Design review of the part built by this model. Coordinates are the model's own, in mm. Face numbers are marked on the shaded views. A direction names the side the tool comes from. Give positions to 0.01 mm unless a question says otherwise; leave off trailing zeros. Loops run counter-clockwise (first coordinate to the right, second up) from the corner with the lowest first, then second, coordinate; pieces in that order, holes last. Notation, with made-up numbers: M 28,34.5 L 57,34.5 A18 cw 57,58.5 Z; hole C 86.25,20.25 d4. An arc over 180 degrees is marked long. Use a Markdown table: item, result. Add a question column.
(1) Add section B-B, the plane z = 14.5. Give the boundary of the cut face in (x, y).
(2) For probe 1 along Y at (x, z) = (0, -5.75); probe 2 along Z at (x, y) = (6.5, -4.5); probe 3 along Z at (x, y) = (-14, -14), list the stretches that pass through material, from the lowest coordinate up.
(3) For the marked faces 1 and 2, list the 3-axis set-ups (+Z, -Z, +X, -X, +Y, -Y) from which the entire face can be reached by the end or side of a thin tool; tool diameter is ignored.
(4) Add section A-A, the plane z = -67. Give the boundary of the cut face in (x, y).
(5) Insertion check: pin 1 Ø1.2 at (x, y) = (0.5, -16.5) entering from +Z; pin 2 Ø8 at (x, z) = (6, -122.5) entering from +Y; pin 3 Ø2.5 at (x, y) = (-16, 0) entering from -Z. Each pin has a flat end and moves straight along its axis. Give the tip position at first contact, or say it passes through.
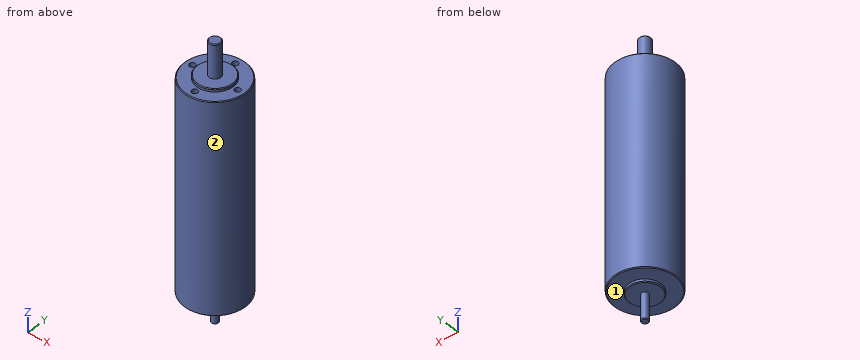
```python
from build123d import *

# Parameters (mm, degrees)
ESQUISSE1_R          = 21
BASE_EXTRUSION_DEPTH = 143.5
ESQUISSE2_R          = 12.5
BOSS_EXTRU_1_DEPTH   = 2
ESQUISSE3_R          = 4
BOSS_EXTRU_2_DEPTH   = 23
ESQUISSE4_R          = 11
BOSS_EXTRU_3_DEPTH   = 2
ESQUISSE5_R          = 2.5
BOSS_EXTRU_4_DEPTH   = 18
CHANFREIN1_SIZE      = 0.5
SKETCH1_R            = 2
EXTRUDE1_DEPTH       = 10


with BuildPart() as part:
    # Esquisse1 → Base-Extrusion (new body)
    with BuildSketch(Plane.XY):
        Circle(ESQUISSE1_R)
    extrude(amount=-BASE_EXTRUSION_DEPTH)

    # Esquisse2 → Boss.-Extru.1 (add)
    with BuildSketch(Plane.XY):
        Circle(ESQUISSE2_R)
    extrude(amount=BOSS_EXTRU_1_DEPTH)

    # Esquisse3 → Boss.-Extru.2 (add)
    with BuildSketch(Plane.XY.offset(2)):
        Circle(ESQUISSE3_R)
    extrude(amount=BOSS_EXTRU_2_DEPTH)

    # Esquisse4 → Boss.-Extru.3 (add)
    with BuildSketch(Plane(origin=(0, 0, -143.5), x_dir=(-1, 0, 0), z_dir=(0, 0, -1))):
        with Locations(Location((0, 0, 0), (0, 0, 180))):
            Circle(ESQUISSE4_R)
    extrude(amount=BOSS_EXTRU_3_DEPTH)

    # Esquisse5 → Boss.-Extru.4 (add)
    with BuildSketch(Plane(origin=(0, 0, -145.5), x_dir=(-1, 0, 0), z_dir=(0, 0, -1))):
        Circle(ESQUISSE5_R)
    extrude(amount=BOSS_EXTRU_4_DEPTH)

    # Chanfrein1
    chanfrein1_edges = [part.edges().sort_by_distance(p)[0] for p in [
        (-11, 0, -145.5),
        (2.5, 0, -163.5),
        (-21, 0, 0),
        (-21, 0, -143.5),
        (-12.5, 0, 2),
        (-4, 0, 25),
    ]]
    chamfer(chanfrein1_edges, length=CHANFREIN1_SIZE)

    # Sketch1 → Extrude1 (cut)
    with BuildSketch(Plane.XY):
        with Locations((0, 16)):
            Circle(SKETCH1_R)
        with Locations((16, 0)):
            Circle(SKETCH1_R)
        with Locations((0, -16)):
            Circle(SKETCH1_R)
        with Locations((-16, 0)):
            Circle(SKETCH1_R)
    extrude(amount=-EXTRUDE1_DEPTH, mode=Mode.SUBTRACT)


solid = part.part
```
Established:
| question | item | result |
|---|---|---|
| 1 | outline | C 0,0 d8 |
| 2 | probe 1 | -21 to -18, -14 to 14, 18 to 21 |
| 2 | probe 2 | -145.5 to 2 |
| 2 | probe 3 | -143.5 to 0 |
| 3 | face 1 | -Z |
| 3 | face 2 | +Z, -Z |
| 4 | outline | C 0,0 d42 |
| 5 | pin 1 | z = -10 |
| 5 | pin 2 | y = 20.9 |
| 5 | pin 3 | z = -143.5 |
